Model file for the job. Use its own axes, mm. Coordinates: 2 decimals unless noted, no trailing zeros. Order: outer loops, then holes, each group sorted by start corner. A loop starts at its lowest first (then second) coordinate and runs counter-clockwise, first axis right, second up. Notation, with made-up numbers: M 83,67.5 L 92,67.5 A30 cw 92,99.5 Z; hole C 21,77 d4. An arc over 180 degrees is marked long. Return JSON: item names as keys, results as strings.
Autodesk Inventor part; units mm, degrees
ref_plane "YZ Plane" through (0, 0, 0) normal (1, 0, 0) x (0, 1, 0)
ref_plane "XZ Plane" through (0, 0, 0) normal (0, 1, 0) x (-1, 0, 0)
ref_plane "XY Plane" through (0, 0, 0) normal (0, 0, 1) x (1, 0, 0)
sketch "スケッチ1" plane through (0, 0, 0) normal (0, 0, 1) x (1, 0, 0)
  line L0 (-55, -170) -> (55, -170)
  line L1 (55, -170) -> (55, 170)
  line L2 (55, 170) -> (-55, 170)
  line L3 (-55, 170) -> (-55, -170)
  line L4 (-55, -170) -> (55, 170) construction
  line L5 (55, -170) -> (-55, 170) construction
  line L6 (-55, 140) -> (-50, 140) construction
  line L7 (-50, 140) -> (-25, 165) construction
  line L8 (-25, 165) -> (-25, 170) construction
  line L9 (-46, 40.5) -> (46, 40.5) construction
  line L10 (46, 40.5) -> (46, 132.5) construction
  line L11 (46, 132.5) -> (-46, 132.5) construction
  line L12 (-46, 132.5) -> (-46, 40.5) construction
  line L13 (-46, 40.5) -> (46, 132.5) construction
  line L14 (46, 40.5) -> (-46, 132.5) construction
  line L15 (-46, 1.5) -> (46, 1.5) construction
  line L16 (46, 1.5) -> (46, 37.5) construction
  line L17 (46, 37.5) -> (-46, 37.5) construction
  line L18 (-46, 37.5) -> (-46, 1.5) construction
  line L19 (-46, 1.5) -> (46, 37.5) construction
  line L20 (46, 1.5) -> (-46, 37.5) construction
  line L21 (0, 0) -> (0, 86.5) construction
  circle A0 centre (0, 86.5) radius 53 construction
  line L22 (-44.7, 41.8) -> (44.7, 41.8) construction
  line L23 (44.7, 41.8) -> (44.7, 131.2) construction
  line L24 (44.7, 131.2) -> (-44.7, 131.2) construction
  line L25 (-44.7, 131.2) -> (-44.7, 41.8) construction
  line L26 (-44.7, 41.8) -> (44.7, 131.2) construction
  line L27 (44.7, 41.8) -> (-44.7, 131.2) construction
  arc A1 (-28.4765, 131.2) -> (-44.7, 114.9765) centre (0, 86.5) ccw
  arc A2 (-44.7, 58.0235) -> (-28.4765, 41.8) centre (0, 86.5) ccw
  arc A3 (28.4765, 41.8) -> (44.7, 58.0235) centre (0, 86.5) ccw
  arc A4 (44.7, 114.9765) -> (28.4765, 131.2) centre (0, 86.5) ccw
  line L28 (-28.4765, 131.2) -> (28.4765, 131.2)
  line L29 (-44.7, 114.9765) -> (-44.7, 58.0235)
  line L30 (-28.4765, 41.8) -> (28.4765, 41.8)
  line L31 (44.7, 58.0235) -> (44.7, 114.9765)
  line L32 (-41.25, 45.25) -> (41.25, 45.25) construction
  line L33 (41.25, 45.25) -> (41.25, 127.75) construction
  line L34 (41.25, 127.75) -> (-41.25, 127.75) construction
  line L35 (-41.25, 127.75) -> (-41.25, 45.25) construction
  line L36 (-41.25, 45.25) -> (41.25, 127.75) construction
  line L37 (41.25, 45.25) -> (-41.25, 127.75) construction
  circle A5 centre (-41.25, 127.75) radius 2.25
  circle A6 centre (-41.25, 45.25) radius 2.25
  circle A7 centre (41.25, 45.25) radius 2.25
  circle A8 centre (41.25, 127.75) radius 2.25
  circle A9 centre (-45, 160) radius 2.25
  circle A10 centre (45, 160) radius 2.25
  circle A11 centre (45, -160) radius 2.25
  circle A12 centre (-45, -160) radius 2.25
  circle A13 centre (-45, 0) radius 2.25 construction
  circle A14 centre (45, 0) radius 2.25 construction
  line L38 (-55, 0) -> (55, 0) construction
  circle A15 centre (-41.25, -49.75) radius 2.25
  arc A16 (-44.7, -36.9765) -> (-28.4765, -53.2) centre (0, -8.5) ccw
  line L39 (-28.4765, -53.2) -> (28.4765, -53.2)
  arc A17 (28.4765, -53.2) -> (44.7, -36.9765) centre (0, -8.5) ccw
  circle A18 centre (41.25, -49.75) radius 2.25
  line L40 (44.7, -36.9765) -> (44.7, 19.9765)
  circle A19 centre (41.25, 32.75) radius 2.25
  arc A20 (44.7, 19.9765) -> (28.4765, 36.2) centre (0, -8.5) ccw
  line L41 (-28.4765, 36.2) -> (28.4765, 36.2)
  circle A21 centre (-41.25, 32.75) radius 2.25
  arc A22 (-28.4765, 36.2) -> (-44.7, 19.9765) centre (0, -8.5) ccw
  line L42 (-44.7, 19.9765) -> (-44.7, -36.9765)
  circle A23 centre (-41.25, -144.75) radius 2.25
  arc A24 (-44.7, -131.9765) -> (-28.4765, -148.2) centre (0, -103.5) ccw
  line L43 (-28.4765, -148.2) -> (28.4765, -148.2)
  arc A25 (28.4765, -148.2) -> (44.7, -131.9765) centre (0, -103.5) ccw
  circle A26 centre (41.25, -144.75) radius 2.25
  line L44 (44.7, -131.9765) -> (44.7, -75.0235)
  circle A27 centre (41.25, -62.25) radius 2.25
  arc A28 (44.7, -75.0235) -> (28.4765, -58.8) centre (0, -103.5) ccw
  line L45 (-28.4765, -58.8) -> (28.4765, -58.8)
  circle A29 centre (-41.25, -62.25) radius 2.25
  arc A30 (-28.4765, -58.8) -> (-44.7, -75.0235) centre (0, -103.5) ccw
  line L46 (-44.7, -75.0235) -> (-44.7, -131.9765)
  point P0 (0, 19.5)
  point P1 (0, 19.5)
  dimension "d12" = 106
  dimension "d0" = 110
  dimension "d1" = 340
  dimension "d2" = 135
  dimension "d3" = 30
  dimension "d4" = 30
  dimension "d5" = 5
  dimension "d6" = 92
  dimension "d7" = 92
  dimension "d8" = 92
  dimension "d9" = 36
  dimension "d10" = 3
  dimension "d11" = 1.5
  dimension "d13" = 89.4
  dimension "d14" = 89.4
  dimension "d15" = 82.5
  dimension "d16" = 82.5
  dimension "d17" = 4.5
  dimension "d25" = 4.5
  dimension "d26" = 10
  dimension "d27" = 10
  dimension "d28" = 10
  dimension "d29" = 10
  dimension "d30" = 10
  dimension "d31" = 10
  dimension "d32" = 10
  dimension "d33" = 10
  dimension "d34" = 10
  dimension "d35" = 10
  dimension "d45" = 95
extrude "押し出し1" add sketch "スケッチ1" along normal blind 3 contours L3 L2 L1 L0 | A15 | L42 A22 L41 A20 L40 A17 L39 A16 | A18 | A19 | A21 | A23 | L46 A30 L45 A28 L44 A25 L43 A24 | A26 | A27 | A29
sketch "スケッチ2" plane through (0, 0, 3) normal (0, 0, 1) x (1, 0, 0)
  circle A0 centre (-45, 160) radius 2.25 construction
  circle A1 centre (45, -160) radius 2.25 construction
  circle A2 centre (-45, -160) radius 2.25 construction
  circle A3 centre (-43, 158) radius 2.75 construction
  line L0 (55, 170) -> (-55, 170)
  line L1 (-55, 170) -> (-55, -170)
  line L2 (-43.7153, 161.8472) -> (-41.4298, 160.2577)
  line L3 (-45.2577, 156.4298) -> (-46.8472, 158.7153)
  circle A4 centre (-45, 160) radius 2.25 construction
  arc A5 (-43.7153, 161.8472) -> (-46.8472, 158.7153) centre (-45, 160) ccw
  arc A6 (-45.2577, 156.4298) -> (-41.4298, 160.2577) centre (-43, 158) ccw
  line L4 (55, 170) -> (-55, 170) construction
  line L5 (0, 170) -> (0, -170) construction
  line L6 (-55, -170) -> (55, -170) construction
  line L7 (-55, 0) -> (55, 0) construction
  line L8 (55, -170) -> (55, 170) construction
  circle A7 centre (45, 160) radius 2.25 construction
  circle A8 centre (43, 158) radius 2.75 construction
  line L9 (43.7153, 161.8472) -> (41.4298, 160.2577)
  line L10 (45.2577, 156.4298) -> (46.8472, 158.7153)
  circle A9 centre (45, 160) radius 2.25 construction
  arc A10 (46.8472, 158.7153) -> (43.7153, 161.8472) centre (45, 160) ccw
  arc A11 (41.4298, 160.2577) -> (45.2577, 156.4298) centre (43, 158) ccw
  circle A12 centre (-45, -160) radius 2.25 construction
  circle A13 centre (-43, -158) radius 2.75 construction
  line L11 (-43.7153, -161.8472) -> (-41.4298, -160.2577)
  line L12 (-45.2577, -156.4298) -> (-46.8472, -158.7153)
  circle A14 centre (-45, -160) radius 2.25 construction
  arc A15 (-46.8472, -158.7153) -> (-43.7153, -161.8472) centre (-45, -160) ccw
  arc A16 (-41.4298, -160.2577) -> (-45.2577, -156.4298) centre (-43, -158) ccw
  circle A17 centre (45, -160) radius 2.25 construction
  line L13 (45.2577, -156.4298) -> (46.8472, -158.7153)
  arc A18 (45.2577, -156.4298) -> (41.4298, -160.2577) centre (43, -158) ccw
  circle A19 centre (43, -158) radius 2.75 construction
  line L14 (43.7153, -161.8472) -> (41.4298, -160.2577)
  circle A20 centre (45, -160) radius 2.25 construction
  arc A21 (43.7153, -161.8472) -> (46.8472, -158.7153) centre (45, -160) ccw
  point P0 (0, 0)
  dimension "d38" = 5.5
  dimension "d39" = 12
  dimension "d40" = 12
extrude "押し出し2" cut sketch "スケッチ2" against normal through all
sketch "スケッチ3" plane through (0, 0, 3) normal (0, 0, 1) x (1, 0, 0)
  line L0 (-55, -170) -> (55, -170) construction
  line L1 (-55, -166.5) -> (55, -166.5)
  line L2 (55, -166.5) -> (55, -170)
  line L3 (55, -170) -> (-55, -170)
  line L4 (-55, -170) -> (-55, -166.5)
  line L5 (-55, -166.5) -> (55, -170) construction
  line L6 (55, -166.5) -> (-55, -170) construction
  line L7 (0, -168.25) -> (0, -170) construction
  point P0 (0, 0)
  dimension "d50" = 3.5
  dimension "d51" = 110
extrude "押し出し3" cut sketch "スケッチ3" against normal through all
equation "\"d4\" = d3"
equation "\"d11\" = 0.5 * d10"
equation "\"d27\" = d26"
equation "\"d28\" = d26"
equation "\"d29\" = d26"
equation "\"d30\" = d26"
equation "\"d31\" = d26"
equation "\"d32\" = d26"
equation "\"d33\" = d26"
equation "\"d34\" = d26"
equation "\"d35\" = d26"
equation "\"d45\" = d7 + d10"
properties part number "bottom_panel" material "アルミニウム 6061"
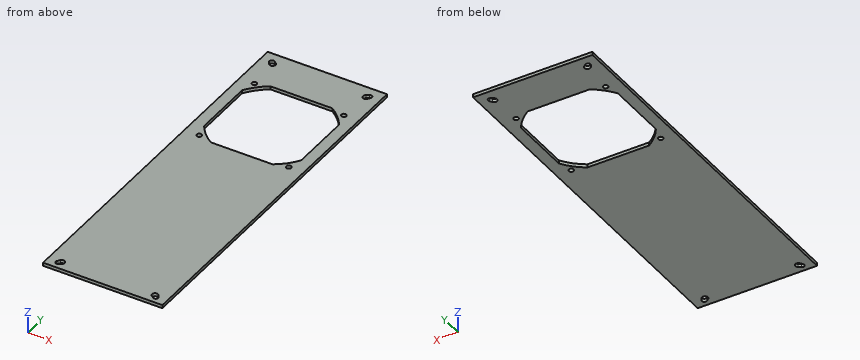
Item 1: Drop a flat-ended pin along its axis: pin 1 Ø3.5 at (x, y) = (41.25, 127.75) entering from +Z. Give the stop position or say it passes through.
Check result:
{"pin 1": "passes through"}
Item 2: Saw through at A-A (x = -8). Write the cut outline in (y, z).
Check result:
{"outline": "M -166.5,0 L 41.8,0 L 41.8,3 L -166.5,3 Z; M 131.2,0 L 170,0 L 170,3 L 131.2,3 Z"}
Item 3: Wall check: line 1 (Y direction, x = 20.5, z = 0.4); line 2 (X direction, y = -158, z = 2); line 3 (Y direction, x = 46.5, z = 1.5). Give the ranges that are in metal, low to high.
Check result:
{"line 1": "y = -166.5 to 41.8, 131.2 to 170", "line 2": "x = -55 to -46.35, -40.25 to 40.25, 46.35 to 55", "line 3": "y = -166.5 to -161.68, -158.22 to 158.22, 161.68 to 170"}
Item 4: Saw through at B-B (z = 2.05). Count the separate pieces of the cut face and the enclosed holes in it, and give its area (3 significant figures).
Check result:
{"separate pieces": "1", "enclosed holes": "9", "area": "29,300 mm2"}
